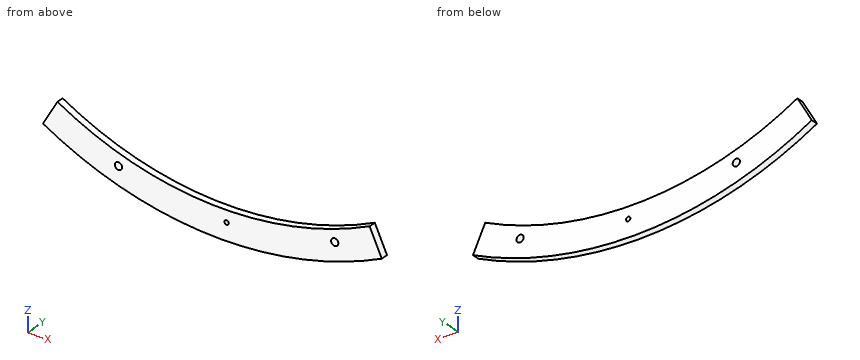
from build123d import *

# Parameters (mm, degrees)
SKETCH1_R           = 254.5
SKETCH1_R_2         = 234.5
BOSS_EXTRUDE1_DEPTH = 5
SKETCH2_W           = 27.805822748
SKETCH2_H           = 60
CUT_EXTRUDE1_DEPTH  = 5
SKETCH3_R           = 2.5
CUT_EXTRUDE2_DEPTH  = 5
SKETCH4_R           = 1.5
CUT_EXTRUDE3_DEPTH  = 5
SKETCH5_W           = 651.212620435
SKETCH5_H           = 357.226439325
CUT_EXTRUDE4_DEPTH  = 10
CUT_EXTRUDE9_START  = -10
SKETCH6_R           = 1.5
SKETCH6_R_2         = 2.5
CUT_EXTRUDE9_DEPTH  = 10
CUT_EXTRUDE10_START = -10
CUT_EXTRUDE10_DEPTH = 10


with BuildPart() as part:
    # Sketch1 → Boss-Extrude1 (new body)
    with BuildSketch(Plane(origin=(0, 0, 0), x_dir=(1, 0, 0), z_dir=(0, 1, 0))):
        with Locations(Location((0, 0, 0), (0, 0, 270))):
            Circle(SKETCH1_R)
        with Locations(Location((0, 0, 0), (0, 0, 270))):
            Circle(SKETCH1_R_2, mode=Mode.SUBTRACT)
    extrude(amount=BOSS_EXTRUDE1_DEPTH)

    # Sketch2 → Cut-Extrude1 (cut)
    with BuildSketch(Plane(origin=(0, 5, 0), x_dir=(1, 0, 0), z_dir=(0, 1, 0))):
        with Locations((-240.597088626, 30)):
            Rectangle(SKETCH2_W, SKETCH2_H)
    cut_extrude1 = extrude(amount=-CUT_EXTRUDE1_DEPTH, mode=Mode.SUBTRACT)

    # Mirror1: Cut-Extrude1 across plane
    add(cut_extrude1.mirror(Plane.XY), mode=Mode.SUBTRACT)

    # Sketch3 → Cut-Extrude2 (cut)
    with BuildSketch(Plane(origin=(0, 5, 0), x_dir=(1, 0, 0), z_dir=(0, 1, 0))):
        with Locations(Location((242.5, 0, 0), (0, 0, 270))):
            Circle(SKETCH3_R)
        with Locations(Location((196.186621136, -142.537923681, 0), (0, 0, 270))):
            Circle(SKETCH3_R)
        with Locations(Location((74.936621136, -230.631205202, 0), (0, 0, 270))):
            Circle(SKETCH3_R)
        with Locations(Location((-74.936621136, -230.631205202, 0), (0, 0, 270))):
            Circle(SKETCH3_R)
        with Locations(Location((-196.186621136, -142.537923681, 0), (0, 0, 270))):
            Circle(SKETCH3_R)
        with Locations((-242.5, 0)):
            Circle(SKETCH3_R)
        with Locations(Location((-196.186621136, 142.537923681, 0), (0, 0, 270))):
            Circle(SKETCH3_R)
        with Locations(Location((-74.936621136, 230.631205202, 0), (0, 0, 270))):
            Circle(SKETCH3_R)
        with Locations(Location((74.936621136, 230.631205202, 0), (0, 0, 270))):
            Circle(SKETCH3_R)
        with Locations(Location((196.186621136, 142.537923681, 0), (0, 0, 270))):
            Circle(SKETCH3_R)
    extrude(amount=-CUT_EXTRUDE2_DEPTH, mode=Mode.SUBTRACT)

    # Sketch4 → Cut-Extrude3 (cut)
    with BuildSketch(Plane(origin=(0, 5, 0), x_dir=(1, 0, 0), z_dir=(0, 1, 0))):
        with Locations(Location((0, -242.5, 0), (0, 0, 270))):
            Circle(SKETCH4_R)
        with Locations(Location((-142.537923681, -196.186621136, 0), (0, 0, 270))):
            Circle(SKETCH4_R)
        with Locations(Location((-230.631205202, -74.936621136, 0), (0, 0, 270))):
            Circle(SKETCH4_R)
        with Locations(Location((-230.631205202, 74.936621136, 0), (0, 0, 270))):
            Circle(SKETCH4_R)
        with Locations(Location((-142.537923681, 196.186621136, 0), (0, 0, 270))):
            Circle(SKETCH4_R)
        with Locations(Location((0, 242.5, 0), (0, 0, 270))):
            Circle(SKETCH4_R)
        with Locations(Location((142.537923681, 196.186621136, 0), (0, 0, 270))):
            Circle(SKETCH4_R)
        with Locations(Location((230.631205202, 74.936621136, 0), (0, 0, 270))):
            Circle(SKETCH4_R)
        with Locations(Location((230.631205202, -74.936621136, 0), (0, 0, 270))):
            Circle(SKETCH4_R)
        with Locations(Location((142.537923681, -196.186621136, 0), (0, 0, 270))):
            Circle(SKETCH4_R)
    extrude(amount=-CUT_EXTRUDE3_DEPTH, mode=Mode.SUBTRACT)

    # Sketch5 → Cut-Extrude4 (cut)
    with BuildSketch(Plane(origin=(0, 5, 0), x_dir=(1, 0, 0), z_dir=(0, 1, 0))):
        with Locations((-71.106310217, -178.613219663)):
            Rectangle(SKETCH5_W, SKETCH5_H)
    extrude(amount=-CUT_EXTRUDE4_DEPTH, mode=Mode.SUBTRACT)

    # Sketch6 → Cut-Extrude9 (cut)
    # profile 1 of 2: a face of its own
    with BuildSketch(Plane(origin=(0, 5, 0), x_dir=(1, 0, 0), z_dir=(0, 1, 0)).offset(CUT_EXTRUDE9_START)):
        with BuildLine():
            Line((-117.25, 203.082957187), (-127.25, 220.403465263))
            ThreePointArc((-127.25, 220.403465263), (-203.737945948, 152.51589878), (-247.326201604, 60))
            Line((-247.326201604, 60), (-226.694177252, 60))
            ThreePointArc((-226.694177252, 60), (-186.259449225, 142.469883043), (-117.25, 203.082957187))
        make_face()
        with Locations((-230.631205202, 74.936621136)):
            Circle(SKETCH6_R, mode=Mode.SUBTRACT)
        with Locations((-196.186621136, 142.537923681)):
            Circle(SKETCH6_R_2, mode=Mode.SUBTRACT)
        with Locations((-142.537923681, 196.186621136)):
            Circle(SKETCH6_R, mode=Mode.SUBTRACT)
    # profile 2 of 2: a face of its own
    with BuildSketch(Plane(origin=(0, 5, 0), x_dir=(1, 0, 0), z_dir=(0, 1, 0)).offset(CUT_EXTRUDE9_START)):
        with BuildLine():
            Line((-254.5, 0), (0, 0))
            Line((0, 0), (-117.25, 203.082957187))
            ThreePointArc((-117.25, 203.082957187), (-186.259449225, 142.469883043), (-226.694177252, 60))
            Line((-226.694177252, 60), (-247.326201604, 60))
            ThreePointArc((-247.326201604, 60), (-252.700186296, 30.213669851), (-254.5, 0))
        make_face()
    extrude(amount=CUT_EXTRUDE9_DEPTH, mode=Mode.SUBTRACT)

    # Sketch7 → Cut-Extrude10 (cut)
    with BuildSketch(Plane(origin=(0, 5, 0), x_dir=(1, 0, 0), z_dir=(0, 1, 0)).offset(CUT_EXTRUDE10_START)):
        with BuildLine():
            Line((254.5, 0), (0, 0))
            Line((0, 0), (107.556347613, 230.655331801))
            ThreePointArc((107.556347613, 230.655331801), (214.643122959, 136.742750324), (254.5, 0))
        make_face()
    extrude(amount=CUT_EXTRUDE10_DEPTH, mode=Mode.SUBTRACT)


solid = part.part
Check sheet for the modelled part. Datum: model origin and axes. Units: mm. Round coordinates to 2 decimals unless told otherwise and drop trailing zeros. Loops run counter-clockwise (first coordinate to the right, second up) from the corner with the lowest first, then second, coordinate; pieces in that order, holes last. Notation, with made-up numbers: M 24,81.5 L 39,81.5 A22 ccw 39,91.5 Z; hole C 43,85 d6. An arc over 180 degrees is marked long. One line per question, with ' | ' between items. Start each with the question number.
Item 1: Scan lines: probe 1 along X at (y, z) = (3.65, -214); probe 2 along Z at (x, y) = (-15.5, 0.5); probe 3 along Z at (x, y) = (92, 3.35). Record each from-to range of solid material in increasing order.
Item 2: Section check C-C (z = -225). Record the boundary of the cut face in (x, y).
Item 3: Section check B-B (y = 2.35). Record the boundary of the cut face in (x, z).
Item 4: Section check A-A (z = -216.5). Record the boundary of the cut face in (x, y).
Item 5: Section check D-D (x = -15). Record the boundary of the cut face in (y, z), and give its area (3 significant figures).
Item 6: Gauge pin test, flat ends, axial feed: pin 1 Ø1.5 at (y, z) = (3, -236.5) entering from -X; pin 2 Ø4 at (x, z) = (-74.94, -230.63) entering from +Y. Record the tip position at first contact, or that the pin passes through.
Worked out:
1) probe 1: -123.55 to -95.89, 95.89 to 99.79 | probe 2: -254.03 to -233.99 | probe 3: -237.29 to -215.7
2) outline: M -118.93,0 L -66.07,0 L -66.07,5 L -118.93,5 Z; M 66.07,0 L 104.92,0 L 104.92,5 L 66.07,5 Z
3) outline: M -127.25,-220.4 A254.5 ccw 107.56,-230.66 L 99.1,-212.53 A234.5 cw -117.25,-203.08 Z; hole C -74.94,-230.63 d5; hole C 0,-242.5 d3; hole C 74.94,-230.63 d5
4) outline: M -125,0 L -90.1,0 L -90.1,5 L -125,5 Z; M 90.1,0 L 100.96,0 L 100.96,5 L 90.1,5 Z
5) outline: M 0,-254.06 L 5,-254.06 L 5,-234.02 L 0,-234.02 Z | area: 100 mm^2
6) pin 1: x = -95.88 | pin 2: through
